from build123d import *

# Parameters (mm, degrees)
F0_R     = 20
F1_DEPTH = 50
F2_DEPTH = 25


with BuildPart() as f1:
    # F0 (on Front) → F1 (new body)
    with BuildSketch(Plane.XZ):
        with BuildLine():
            ThreePointArc((-36.518415, 16.321929), (-8.344561, -39.119922), (40, 0))
            ThreePointArc((40, 0), (39.119922, 8.344561), (36.518415, 16.321929))
            ThreePointArc((36.518415, 16.321929), (0, 40), (-36.518415, 16.321929))
        make_face()
        Circle(F0_R, mode=Mode.SUBTRACT)
    extrude(amount=F1_DEPTH)

    # F0 (on Front) → F2 (join)
    with BuildSketch(Plane.XZ):
        with BuildLine():
            ThreePointArc((-36.518415, 16.321929), (0, 40), (36.518415, 16.321929))
            Line((36.518415, 16.321929), (16.116004, 61.969948))
            ThreePointArc((16.116004, 61.969948), (0, 72.419358), (-16.116004, 61.969948))
            Line((-16.116004, 61.969948), (-36.518415, 16.321929))
        make_face()
    extrude(amount=F2_DEPTH)


solid = f1.part
Can you work these out from the model? Positions are in its coordinate system, mm. Round coordinates to 2 decimals unless told otherwise and drop trailing zeros. Loops run counter-clockwise (first coordinate to the right, second up) from the corner with the lowest first, then second, coordinate; pieces in that order, holes last. Notation, with made-up numbers: (40, -2) - (51, -2) arc R17 ccw to (51, 7) - close; hole circle Ø7 at (79.25, 10.25). An arc over 180 degrees is marked (long way). Answer in a Markdown table with one row per item. Add a question column.
Q1. I want a section at A-A on x = 0. List the corners of the cut face in (y, z) for me, and give its area (3 significant figures).
Q2. We'd pull the mould along Z, two halves only. Please class faces 1 (the flat face through (0, -25, 53)), 2 (the cylindrical face through (-4.336, -24.65, -19.524)), 3 (the cylindrical face through (0.284, -12.325, 72.417)): pulls with the +Z half, pulls with the -Z half, needs draft (parallel to the pull), parting line crosses it, or undercut.
Q3. I want a section at D-D on z = 38. List the corners of the cut face in (x, y) for me.
Q4. For pin 1 Ø1.5 at (x, y) = (-27, -23) entering from -Z; pin 2 Ø8 at (x, y) = (-11, -17) entering from +Z; pin 3 Ø1.5 at (y, z) = (-45, 6.5) entering from +X, each with a flat end and sliding along its axis, tell me the tip position at first contact or that it passes through.
Q5. I want a section at B-B on z = -4. List the corners of the cut face in (x, y) for me.
Q6. I want a section at C-C on y = -23.5. List the corners of the cut face in (x, z) for me.
Q7. I need wall thicknesses on L1, parallel to Z at x = 0, y = -13.5; L2, parallel to X at y = -17, z = 0.5; L3, parallel to Z at x = 0, y = -39. Which ranges of each line are inside material? Lowest first, please.
A:
| question | item | result |
|---|---|---|
| 1 | outline | (-50, -40) - (0, -40) - (0, -20) - (-50, -20) - close; (-50, 20) - (0, 20) - (0, 72.42) - (-25, 72.42) - (-25, 40) - (-50, 40) - close |
| 1 | area | 2,810 mm^2 |
| 2 | face 1 | needs draft |
| 2 | face 2 | undercut |
| 2 | face 3 | pulls with the +Z half |
| 3 | outline | (-26.83, -25) - (-12.49, -25) - (-12.49, -50) - (12.49, -50) - (12.49, -25) - (26.83, -25) - (26.83, 0) - (-26.83, 0) - close |
| 4 | pin 1 | z = -30.18 |
| 4 | pin 2 | z = 70.97 |
| 4 | pin 3 | x = 39.58 |
| 5 | outline | (-39.8, -50) - (-19.6, -50) - (-19.6, 0) - (-39.8, 0) - close; (19.6, -50) - (39.8, -50) - (39.8, 0) - (19.6, 0) - close |
| 6 | outline | (-36.52, 16.32) arc R40 ccw (long way) to (40, 0) arc R40 ccw to (36.52, 16.32) - (16.12, 61.97) arc R17.65 ccw to (-16.12, 61.97) - close; hole circle Ø40 at (0, 0) |
| 7 | L1 | -40 to -20, 20 to 72.42 |
| 7 | L2 | -40 to -19.99, 19.99 to 40 |
| 7 | L3 | -40 to -20, 20 to 40 |
